Geometry: final body of the model. Coordinates: model frame, mm. A direction names the side the tool comes from. Give positions to 0.01 mm unless a question says otherwise; leave off trailing zeros. Write each loop counter-clockwise with the first axis right and the second up, starting at its lowest first coordinate (ties: lowest second). Pieces come first, ordered by that corner, then holes. Notation, with made-up numbers: M 3,-26 L 10,-26 A13 cw 10,-9 Z; hole C 58,73 d9. An arc over 180 degrees is marked long. Use a Markdown table: item, result. Add a question column.
(1) Cut plane C-C (x = 9). Output: boundary loops of the cut face in (y, z), plus the area to 3 significant figures.
(2) Pin query (flat end, axial travel): pin 1 Ø1 at (x, y) = (-49.5, 16.5) entering from -Z; pin 2 Ø1.8 at (x, y) = (51, 13) entering from +Z; pin 3 Ø3 at (x, y) = (-51.5, 14) entering from +Z; pin 4 Ø1.8 at (x, z) = (40, 22.5) entering from +Y. Return the tip coordinate at first contact, or that it passes through.
(3) Cut plane A-A (y = 13.75). Output: boundary loops of the cut face in (x, z).
(4) Material intervals for L1, parallel to Z at x = -43, y = 14.25; L2, parallel to Z at x = -16.5, y = 16.25; L3, parallel to X at y = 5.25, z = 22.5, sorted ascending.
(5) Cut plane D-D (z = 14). Output: boundary loops of the cut face in (x, y).
(6) Draft query along Z for faces 1 (the cylindrical face through (-47.196, 8.916, 29.789)), 2 (the cylindrical face through (-48.789, 16.479, 31.196)), 3 (the cylindrical face through (48.696, 16.479, -31.289)), 4 (the flat face through (-49, 8, 0)). Return one class per face: released by +Z, released by -Z, zero draft, split by the parting line, or undercut.
(7) Cut plane B-B (z = -1). Output: boundary loops of the cut face in (x, y), plus the area to 3 significant figures.
(8) Reachability of faces 5 (the flat face through (50, 16, -9.737)), 6 (the flat face through (34.809, 16, 32)), 7 (the cylindrical face through (-46.696, 16.479, -29.289)) from +Z, -Z, +X, -X, +Y, -Y: full face, straight path, thin tool, end or side. Return the list, or none.
```python
from build123d import *

# Parameters (mm, degrees)
SKETCH1_W           = 105
SKETCH1_H           = 70
BOSS_EXTRUDE1_DEPTH = 15
SKETCH3_W           = 98
SKETCH3_H           = 63
CUT_EXTRUDE1_DEPTH  = 12
FILLET1_R           = 6
SKETCH4_R           = 3.5
BOSS_EXTRUDE2_DEPTH = 5
SKETCH5_R           = 1
CUT_EXTRUDE2_DEPTH  = 8
SKETCH6_W           = 3.5
SKETCH6_H           = 18.3
SKETCH6_W_2         = 14
SKETCH6_H_2         = 3.5
SKETCH6_H_3         = 20
CUT_EXTRUDE3_DEPTH  = 6
BOSS_EXTRUDE3_DEPTH = 3


with BuildPart() as part:
    # Sketch1 → Boss-Extrude1 (new body)
    with BuildSketch(Plane(origin=(0, 0, 0), x_dir=(1, 0, 0), z_dir=(0, 1, 0))):
        Rectangle(SKETCH1_W, SKETCH1_H)
    extrude(amount=BOSS_EXTRUDE1_DEPTH)

    # Sketch3 → Cut-Extrude1 (cut)
    with BuildSketch(Plane(origin=(0, 15, 0), x_dir=(1, 0, 0), z_dir=(0, 1, 0))):
        Rectangle(SKETCH3_W, SKETCH3_H)
    extrude(amount=-CUT_EXTRUDE1_DEPTH, mode=Mode.SUBTRACT)

    # Fillet1
    fillet1_edges = [part.edges().sort_by_distance(p)[0] for p in [
        (-49, 9, 31.5),
        (-49, 9, -31.5),
        (49, 9, -31.5),
        (49, 9, 31.5),
        (52.5, 7.5, 35),
        (-52.5, 7.5, 35),
        (-52.5, 7.5, -35),
        (52.5, 7.5, -35),
    ]]
    fillet(fillet1_edges, radius=FILLET1_R)

    # Sketch4 → Boss-Extrude2 (add)
    with BuildSketch(Plane(origin=(0, 3, 0), x_dir=(1, 0, 0), z_dir=(0, 1, 0))):
        with Locations(Location((40, -22.5, 0), (0, 0, 270))):
            Circle(SKETCH4_R)
        with Locations(Location((40, 19.2, 0), (0, 0, 270))):
            Circle(SKETCH4_R)
        with Locations(Location((-36.1, -22.5, 0), (0, 0, 270))):
            Circle(SKETCH4_R)
        with Locations(Location((-36.1, 19.2, 0), (0, 0, 270))):
            Circle(SKETCH4_R)
    extrude(amount=BOSS_EXTRUDE2_DEPTH)

    # Sketch5 → Cut-Extrude2 (cut)
    with BuildSketch(Plane(origin=(0, 8, 0), x_dir=(1, 0, 0), z_dir=(0, 1, 0))):
        with Locations(Location((-36.1, 19.2, 0), (0, 0, 270))):
            Circle(SKETCH5_R)
        with Locations(Location((-36.1, -22.5, 0), (0, 0, 270))):
            Circle(SKETCH5_R)
        with Locations(Location((40, -22.5, 0), (0, 0, 270))):
            Circle(SKETCH5_R)
        with Locations(Location((40, 19.06026255, 0), (0, 0, 270))):
            Circle(SKETCH5_R)
    extrude(amount=-CUT_EXTRUDE2_DEPTH, mode=Mode.SUBTRACT)

    # Sketch6 → Cut-Extrude3 (cut)
    with BuildSketch(Plane(origin=(0, 15, 0), x_dir=(1, 0, 0), z_dir=(0, 1, 0))):
        with Locations((50.75, 0.51)):
            Rectangle(SKETCH6_W, SKETCH6_H)
        with Locations((27.76, -33.25)):
            Rectangle(SKETCH6_W_2, SKETCH6_H_2)
        with Locations((-50.75, 0)):
            Rectangle(SKETCH6_W, SKETCH6_H_3)
    extrude(amount=-CUT_EXTRUDE3_DEPTH, mode=Mode.SUBTRACT)

    # Sketch7 → Boss-Extrude3 (add)
    with BuildSketch(Plane(origin=(0, 15, 0), x_dir=(1, 0, 0), z_dir=(0, 1, 0))):
        with BuildLine():
            Line((-44.5, 33), (44.5, 33))
            ThreePointArc((44.5, 33), (48.742640687, 31.242640687), (50.5, 27))
            Line((50.5, 27), (50.5, 9.736559035))
            Line((50.5, 9.736559035), (48.5, 9.736559035))
            Line((48.5, 9.736559035), (48.5, 25))
            ThreePointArc((48.5, 25), (46.742640687, 29.242640687), (42.5, 31))
            Line((42.5, 31), (-42.5, 31))
            ThreePointArc((-42.5, 31), (-46.742640687, 29.242640687), (-48.5, 25))
            Line((-48.5, 25), (-48.5, 10))
            Line((-48.5, 10), (-50.5, 10))
            Line((-50.5, 10), (-50.5, 27))
            ThreePointArc((-50.5, 27), (-48.742640687, 31.242640687), (-44.5, 33))
        make_face()
        with BuildLine():
            Line((-44.5, -33), (20.754470261, -33))
            Line((20.754470261, -33), (20.754470261, -31))
            Line((20.754470261, -31), (-42.5, -31))
            ThreePointArc((-42.5, -31), (-46.742640687, -29.242640687), (-48.5, -25))
            Line((-48.5, -25), (-48.5, -10.02702289))
            Line((-48.5, -10.02702289), (-50.5, -10.02702289))
            Line((-50.5, -10.02702289), (-50.5, -27))
            ThreePointArc((-50.5, -27), (-48.742640687, -31.242640687), (-44.5, -33))
        make_face()
        with BuildLine():
            Line((50.5, -8.739580153), (50.5, -27))
            ThreePointArc((50.5, -27), (48.742640687, -31.242640687), (44.5, -33))
            Line((44.5, -33), (34.809182833, -33))
            Line((34.809182833, -33), (34.809182833, -31))
            Line((34.809182833, -31), (42.5, -31))
            ThreePointArc((42.5, -31), (46.742640687, -29.242640687), (48.5, -25))
            Line((48.5, -25), (48.5, -8.739580153))
            Line((48.5, -8.739580153), (50.5, -8.739580153))
        make_face()
    extrude(amount=BOSS_EXTRUDE3_DEPTH)


solid = part.part
```
Answer list:
| question | item | result |
|---|---|---|
| 1 | outline | M 0,-35 L 15,-35 L 15,-33 L 18,-33 L 18,-31 L 15,-31 L 15,-31.5 L 3,-31.5 L 3,31.5 L 15,31.5 L 15,31 L 18,31 L 18,33 L 15,33 L 15,35 L 0,35 Z |
| 1 | area | 306 mm² |
| 2 | pin 1 | z = -30.97 |
| 2 | pin 2 | z = 33.8 |
| 2 | pin 3 | z = 33.87 |
| 2 | pin 4 | through |
| 3 | outline | M -52.5,-29 A6 ccw -46.5,-35 L 46.5,-35 A6 ccw 52.5,-29 L 52.5,-9.66 L 49,-9.66 L 49,-25.5 A6 cw 43,-31.5 L -43,-31.5 A6 cw -49,-25.5 L -49,-10 L -52.5,-10 Z; M -52.5,10 L -49,10 L -49,25.5 A6 cw -43,31.5 L 20.76,31.5 L 20.76,35 L -46.5,35 A6 ccw -52.5,29 Z; M 34.76,31.5 L 43,31.5 A6 cw 49,25.5 L 49,8.64 L 52.5,8.64 L 52.5,29 A6 ccw 46.5,35 L 34.76,35 Z |
| 4 | L1 | -35 to -31.5, 31.5 to 35 |
| 4 | L2 | -33 to -31, 31 to 33 |
| 4 | L3 | -52.5 to -49, -39.6 to -37.1, -35.1 to -32.6, 36.5 to 39, 41 to 43.5, 49 to 52.5 |
| 5 | outline | M -52.5,0 L 52.5,0 L 52.5,15 L 50.5,15 L 50.5,18 L 48.5,18 L 48.5,15 L 49,15 L 49,3 L -49,3 L -49,15 L -48.5,15 L -48.5,18 L -50.5,18 L -50.5,15 L -52.5,15 Z |
| 6 | face 1 | undercut |
| 6 | face 2 | released by +Z |
| 6 | face 3 | released by -Z |
| 6 | face 4 | undercut |
| 7 | outline | M -52.5,0 L 52.5,0 L 52.5,9 L 49,9 L 49,3 L -49,3 L -49,9 L -52.5,9 Z |
| 7 | area | 357 mm² |
| 8 | face 5 | +X, -X, +Y |
| 8 | face 6 | +Z, +Y |
| 8 | face 7 | +Y |
